Can you work these out from the drawing? Everything is in mm from the part's minimum corner. A direction names the side the tool comes from. Round coordinates to 2 decimals unless told otherwise and drop trailing zeros. Order: outer loops, then holes, each group sorted by start corner. A loop starts at its lowest first (then second) coordinate and runs counter-clockwise, first axis right, second up. Notation, with made-up numbers: M 52.25,9.25 L 95.25,9.25 A29 ccw 95.25,46.25 Z; hole C -15,72 d7. An arc over 180 degrees is marked long. Answer as CSV lines item,"result". Start each with the question number.
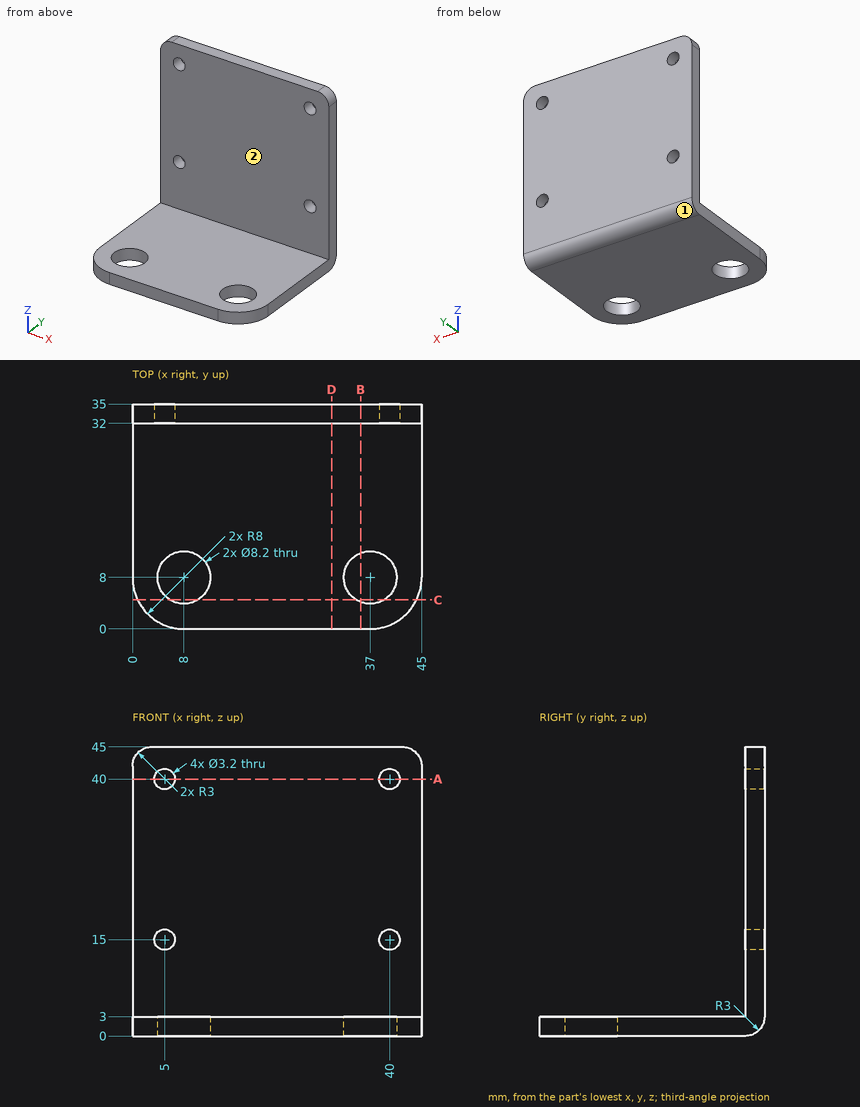
(1) I'm going to push flat-ended pins straight in: P1, Ø4, axis at x = 38.5, y = 23.5, coming from the +Z side; P2, Ø5, axis at x = 27.5, y = 9, coming from the -Z side; P3, Ø12, axis at x = 10, z = 12, coming from the -Y side. Where does each tip first touch, or does it pass through?
(2) For the marked faces 1 and 2, which set-ups out of +Z, -Z, +X, -X, +Y, -Y let a thin tool reach every point of the face, with its end or its side?
(3) I want a section at A-A on z = 40. Write out the boundary of the cut face in (x, y).
(4) If I drill on line 1 along X through (y, z) = (33.4, 15); line 2 along Z through (x, y) = (26, 14.5); line 3 along Y through (x, z) = (37, 29), over which ranges is the centre line in solid material (lowest first)?
(5) I want a section at D-D on x = 31. Write out the boundary of the cut face in (y, z).
(6) I want a section at C-C on y = 4.5. Write out the boundary of the cut face in (x, z), and give its area (3 significant figures).
(7) I want a section at B-B on x = 35.5. Write out the boundary of the cut face in (y, z), and give its area (3 significant figures).
From the geometry:
1,P1,"z = 3"
1,P2,"z = 0"
1,P3,"y = 32"
2,face 1,"-Z, +X, -X, +Y"
2,face 2,"+Z, +X, -X, -Y"
3,outline,"M 0,32 L 3.4,32 L 3.4,35 L 0,35 Z; M 6.6,32 L 38.4,32 L 38.4,35 L 6.6,35 Z; M 41.6,32 L 45,32 L 45,35 L 41.6,35 Z"
4,line 1,"0 to 3.4, 6.6 to 38.4, 41.6 to 45"
4,line 2,"0 to 3"
4,line 3,"32 to 35"
5,outline,"M 0,0 L 32,0 A3 ccw 35,3 L 35,45 L 32,45 L 32,3 L 0,3 Z"
6,outline,"M 0.81,0 L 5.86,0 L 5.86,3 L 0.81,3 Z; M 10.14,0 L 34.86,0 L 34.86,3 L 10.14,3 Z; M 39.14,0 L 44.19,0 L 44.19,3 L 39.14,3 Z"
6,area,"105 mm²"
7,outline,"M 0,0 L 4.18,0 L 4.18,3 L 0,3 Z; M 11.82,0 L 32,0 A3 ccw 35,3 L 35,45 L 32,45 L 32,3 L 11.82,3 Z"
7,area,"206 mm²"
